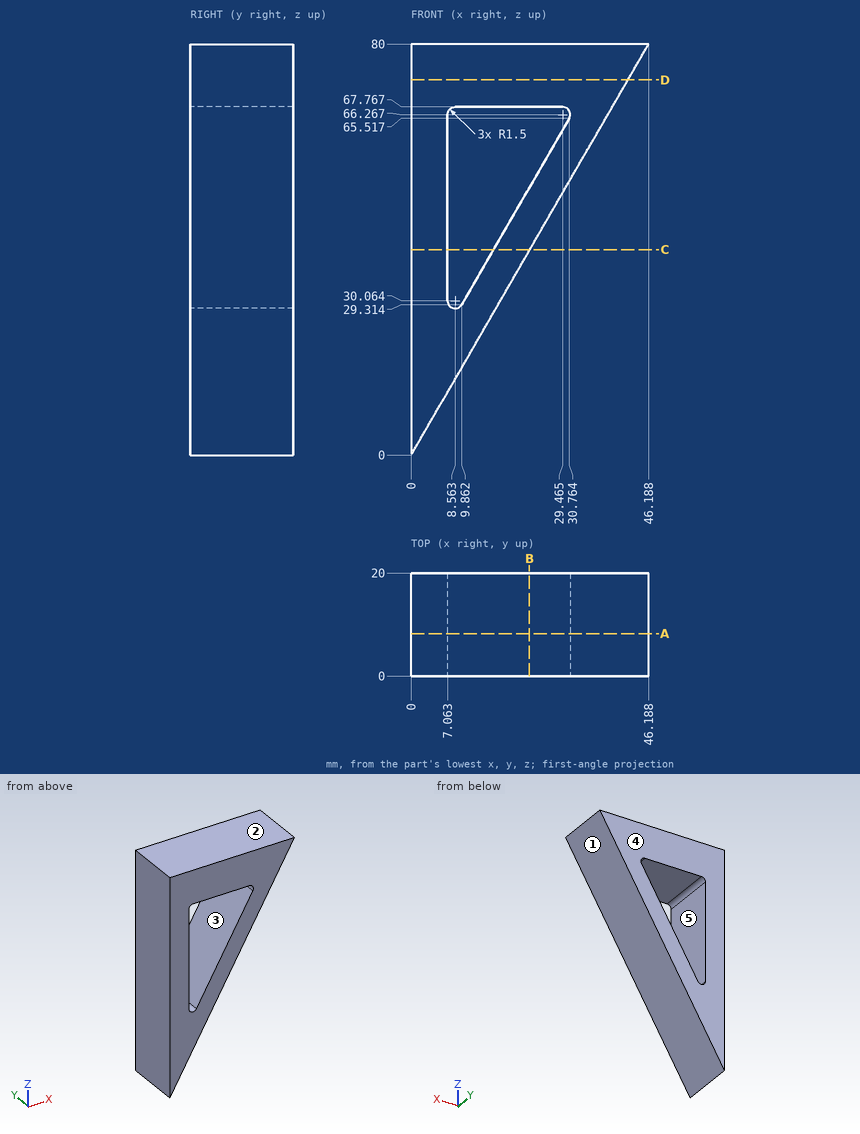
Check sheet for the drawn part. Datum: minimum x, y, z corner. Units: mm. A direction names the side the tool comes from. Coordinates: 2 decimals unless noted, no trailing zeros. Order: outer loops, then holes, each group sorted by start corner. A loop starts at its lowest first (then second) coordinate and runs counter-clockwise, first axis right, second up. Notation, with made-up numbers: M 17.5,-38 L 36.5,-38 A15 cw 36.5,-28 Z; hole C 83,-12.5 d6. An arc over 180 degrees is marked long. One line per item, written item: value. Start each with the question number.
Item 1: Access from +Z, -Z, +X, -X, +Y, -Y to the whole of each face (thin tool, end or side, straight path). Record for the marked faces 4 and 5.
Item 2: Sectioned sample at B-B (x = 23). Enter the section's corners in (y, z), then the cut area to 3 significant figures.
Item 3: Scan lines: probe 1 along Z at (x, y) = (22, 9.25) (1 decimal); probe 2 along Z at (x, y) = (24, 12.5) (1 decimal); probe 3 along X at (y, z) = (14, 41). Record each from-to range of solid material in increasing order.
Item 4: Sectioned sample at C-C (z = 40). Enter the section's corners in (x, y).
Item 5: Mould release check, pull along Z, two halves, no side actions. Record for the marked faces 1, 2 and 3: released by +Z, released by -Z, zero draft, split by the parting line, or undercut.
Item 6: Sectioned sample at D-D (z = 73). Enter the section's corners in (x, y), then the cut area to 3 significant figures.
Item 7: Gauge pin test, flat ends, axial feed: pin 1 (5 mm diameter, centred on x = 12, z = 40.5, fed in from +Y); pin 2 (6 mm diameter, centred on x = 8.5, z = 24, fed in from -Y); pin 3 (5 mm diameter, centred on y = 13.5, z = 49, fed in from +X); pin 4 (10 mm diameter, centred on x = 21, y = 8.5, fed in from -Z) (1 decimal). Record the tip position at first contact, or that the pin passes through.
Item 8: Sectioned sample at A-A (y = 8.25). Enter the section's corners in (x, z) (1 decimal).
Conclusion:
1. face 4: +Z, -Z, +X, -X, +Y
1. face 5: +Y, -Y
2. outline: M 0,39.84 L 20,39.84 L 20,52.07 L 0,52.07 Z; M 0,67.77 L 20,67.77 L 20,80 L 0,80 Z
2. area: 489 mm^2
3. probe 1: z = 38.1 to 50.3, 67.8 to 80
3. probe 2: z = 41.6 to 53.8, 67.8 to 80
3. probe 3: x = 0 to 7.06, 16.61 to 23.67
4. outline: M 0,0 L 7.06,0 L 7.06,20 L 0,20 Z; M 16.03,0 L 23.09,0 L 23.09,20 L 16.03,20 Z
5. face 1: released by -Z
5. face 2: released by +Z
5. face 3: undercut
6. outline: M 0,0 L 42.15,0 L 42.15,20 L 0,20 Z
6. area: 843 mm^2
7. pin 1: passes through
7. pin 2: stops at y = 0
7. pin 3: stops at x = 29.73
7. pin 4: stops at z = 27.7
8. outline: M 0,0 L 46.2,80 L 0,80 Z; hole M 7.1,30.1 A1.5 ccw 9.9,29.3 L 30.8,65.5 A1.5 ccw 29.5,67.8 L 8.6,67.8 A1.5 ccw 7.1,66.3 Z
